Verification items for the finished model (mm, model axes). Give positions to 0.01 mm unless a question says otherwise; leave off trailing zeros. Use CSV: the item, a comma, the result in double quotes. Start each with the question number.
```python
from build123d import *

# Parameters (mm, degrees)
SKETCH1_W           = 76.2
SKETCH1_H           = 12.7
BOSS_EXTRUDE1_DEPTH = 6
CUT_EXTRUDE1_DEPTH  = 3.1
LPATTERN1_START     = 2.9
LPATTERN1_DEPTH     = 3.1
SKETCH3_R           = 0.5
CUT_EXTRUDE2_DEPTH  = 0.5
FILLET1_R           = 6.35
CHAMFER1_SIZE       = 0.5


# Read off the part's stored shape, not the designer's step: LPattern1
with BuildPart() as part:
    # Sketch1 → Boss-Extrude1 (new body)
    with BuildSketch(Plane(origin=(0, 0, 0), x_dir=(1, 0, 0), z_dir=(0, 1, 0))):
        Rectangle(SKETCH1_W, SKETCH1_H)
    extrude(amount=BOSS_EXTRUDE1_DEPTH)

    # Sketch2 → Cut-Extrude1 (cut)
    with BuildSketch(Plane(origin=(0, 6, 0), x_dir=(1, 0, 0), z_dir=(0, 1, 0))):
        Polygon((1.991858429, 3.45), (-1.991858429, 3.45), (-3.983716857, 0), (-1.991858429, -3.45), (1.991858429, -3.45), (3.983716857, 0), align=None)
    extrude(amount=-CUT_EXTRUDE1_DEPTH, mode=Mode.SUBTRACT)

    # LPattern1 outline → LPattern1 (cut)
    with BuildSketch(Plane(origin=(0, 0, 0), x_dir=(1, 0, 0), z_dir=(0, 1, 0)).offset(LPATTERN1_START)):
        Polygon((-8.022575328, -3.425), (-6.045150656, 0), (-8.022575328, 3.425), (-11.977424672, 3.425), (-13.954849344, 0), (-11.977424672, -3.425), align=None)
        Polygon((-18.037009085, -3.4), (-16.07401817, 0), (-18.037009085, 3.4), (-21.962990915, 3.4), (-23.92598183, 0), (-21.962990915, -3.4), align=None)
        Polygon((-28.051442841, -3.375), (-26.102885683, 0), (-28.051442841, 3.375), (-31.948557159, 3.375), (-33.897114317, 0), (-31.948557159, -3.375), align=None)
        Polygon((12.006292185, -3.475), (14.012584371, 0), (12.006292185, 3.475), (7.993707815, 3.475), (5.987415629, 0), (7.993707815, -3.475), align=None)
        Polygon((22.020725942, -3.5), (24.041451884, 0), (22.020725942, 3.5), (17.979274058, 3.5), (15.958548116, 0), (17.979274058, -3.5), align=None)
        Polygon((32.035159699, -3.525), (34.070319398, 0), (32.035159699, 3.525), (27.964840301, 3.525), (25.929680602, 0), (27.964840301, -3.525), align=None)
    extrude(amount=LPATTERN1_DEPTH, mode=Mode.SUBTRACT)

    # Sketch3 → Cut-Extrude2 (cut)
    with BuildSketch(Plane(origin=(0, 6, 0), x_dir=(1, 0, 0), z_dir=(0, 1, 0))):
        with Locations(Location((-35.1, 3.35, 0), (0, 0, 270))):
            Circle(SKETCH3_R)
    extrude(amount=-CUT_EXTRUDE2_DEPTH, mode=Mode.SUBTRACT)

    # Fillet1
    fillet1_edges = [part.edges().sort_by_distance(p)[0] for p in [
        (38.1, 3, -6.35),
        (38.1, 3, 6.35),
        (-38.1, 3, -6.35),
        (-38.1, 3, 6.35),
    ]]
    fillet(fillet1_edges, radius=FILLET1_R - 0.0001)  # a hair under: the kernel refuses the full size

    # Chamfer1
    chamfer1_edges = [part.edges().sort_by_distance(p)[0] for p in [
        (-35.1, 6, -3.85),
        (2.987787643, 6, -1.725),
        (0, 6, -3.45),
        (-2.987787643, 6, -1.725),
        (-2.987787643, 6, 1.725),
        (0, 6, 3.45),
        (2.987787643, 6, 1.725),
        (33.052739548, 6, -1.7625),
        (30, 6, -3.525),
        (26.947260452, 6, -1.7625),
        (26.947260452, 6, 1.7625),
        (30, 6, 3.525),
        (33.052739548, 6, 1.7625),
        (23.031088913, 6, -1.75),
        (20, 6, -3.5),
        (16.968911087, 6, -1.75),
        (16.968911087, 6, 1.75),
        (20, 6, 3.5),
        (23.031088913, 6, 1.75),
        (13.009438278, 6, -1.7375),
        (10, 6, -3.475),
        (6.990561722, 6, -1.7375),
        (6.990561722, 6, 1.7375),
        (10, 6, 3.475),
        (13.009438278, 6, 1.7375),
        (-27.077164262, 6, -1.6875),
        (-30, 6, -3.375),
        (-32.922835738, 6, -1.6875),
        (-32.922835738, 6, 1.6875),
        (-30, 6, 3.375),
        (-27.077164262, 6, 1.6875),
        (-17.055513628, 6, -1.7),
        (-20, 6, -3.4),
        (-22.944486373, 6, -1.7),
        (-22.944486372, 6, 1.7),
        (-20, 6, 3.4),
        (-17.055513627, 6, 1.7),
        (-7.033862992, 6, -1.7125),
        (-10, 6, -3.425),
        (-12.966137008, 6, -1.7125),
        (-12.966137008, 6, 1.7125),
        (-10, 6, 3.425),
        (-7.033862992, 6, 1.7125),
    ]]
    chamfer(chamfer1_edges, length=CHAMFER1_SIZE - 0.0001)  # a hair under: the kernel refuses the full size


solid = part.part
```
(1) Go/stop test with flat-tipped pins: pin 1 (3 mm diameter, centred on y = 1.5, z = -4, fed in from -X); pin 2 (2 mm diameter, centred on y = 3, z = 3, fed in from +X); pin 3 (2 mm diameter, centred on x = -1.5, z = -0.5, fed in from +Y). Record where each tip stops, or that it passes through.
(2) Draft check along Z on faces 1 (the face through (-23.142, 5.747, -1.851)), 2 (the face through (36.19, 3.04, -4.54)), 3 (the face through (3, 4.2, 1.7)). Enter one of: released by +Z, released by -Z, zero draft, split by the parting line, or undercut.
(3) Thickness scan on line 1 (Z direction, x = 30, y = 3.25) (3 decimals); line 2 (Y direction, x = 32.5, z = 0); line 3 (Z direction, x = -3, y = 3). Record the ranges inside material, lowest first. Write a range as from..to.
Data:
1,pin 1,"stops at x = -37.59"
1,pin 2,"stops at x = 37.78"
1,pin 3,"stops at y = 2.9"
2,face 1,"undercut"
2,face 2,"released by -Z"
2,face 3,"undercut"
3,line 1,"z = -6.35..-3.525, 3.525..6.35"
3,line 2,"y = 0..2.9"
3,line 3,"z = -6.35..-1.7, 1.7..6.35"
